The listing builds one solid part. Answer for the finished solid, in the listing's coordinates (mm). A direction names the side the tool comes from. Coordinates: 2 decimals unless noted, no trailing zeros. Order: outer loops, then holes, each group sorted by start corner. A loop starts at its lowest first (then second) coordinate and runs counter-clockwise, first axis right, second up. Notation, with made-up numbers: (44, -10) -> (89, -10) arc R25 ccw to (89, 23) -> close; hole circle Ø10 at (5, 4). An arc over 180 degrees is marked (long way). Answer in a Markdown table with one row per item.
Autodesk Inventor part; units mm, degrees
ref_plane "YZ Plane" through (0, 0, 0) normal (1, 0, 0) x (0, 1, 0)
ref_plane "XZ Plane" through (0, 0, 0) normal (0, 1, 0) x (-1, 0, 0)
ref_plane "XY Plane" through (0, 0, 0) normal (0, 0, 1) x (1, 0, 0)
sketch "Sketch1" plane through (0, 0, 0) normal (0, 0, 1) x (1, 0, 0)
  line L0 (0, 0) -> (12.5, 0)
  line L1 (12.5, 0) -> (12.5, 30)
  line L2 (12.5, 30) -> (17.5, 30)
  line L3 (17.5, 30) -> (17.5, -5)
  line L4 (17.5, -5) -> (-17.5, -5)
  line L5 (-17.5, -5) -> (-17.5, 30)
  line L6 (-17.5, 30) -> (-12.5, 30)
  line L7 (-12.5, 30) -> (-12.5, 0)
  line L8 (-12.5, 0) -> (12.5, 0)
  dimension "d0" = 12.5
  dimension "d1" = 30
  dimension "d2" = 5
  dimension "d3" = 35
  dimension "d4" = 35
  dimension "d5" = 35
  dimension "d6" = 5
  dimension "d8" = 30
extrude "Extrusion1" add sketch "Sketch1" along normal blind 10
sketch "Sketch2" plane through (-17.5, -5, 0) normal (0, -1, 0) x (1, 0, 0)
  line L0 (5, 10) -> (0, 10)
  line L1 (30, 0) -> (35, 0)
  line L2 (0, 10) -> (35, 0)
  circle A0 centre (17.5, 5) radius 3
  point P0 (17.5, 0)
  dimension "d11" = 6
extrude "Extrusion2" add sketch "Sketch2" along normal blind 50
sketch "Sketch3" plane through (-17.5, -5, 0) normal (-1, 0, 0) x (0, 0, 1)
  line L0 (0, 35) -> (10, 35)
  line L1 (5, 35) -> (5, 25)
  circle A0 centre (5, 25) radius 2.5
  point P0 (0, 5)
  dimension "d14" = 10
  dimension "d15" = 5
extrude "Extrusion3" cut sketch "Sketch3" against normal blind 35
properties part number "TopFork"
(1) A cutting plane is placed at A-A, the plane z = 5. Determine the outline of the cut face in (x, y).
Check values:
| item | result |
|---|---|
| outline | (-17.5, -5) -> (-3, -5) -> (-3, -55) -> (3, -55) -> (3, -5) -> (17.5, -5) -> (17.5, 17.5) -> (12.5, 17.5) -> (12.5, 0) -> (-12.5, 0) -> (-12.5, 17.5) -> (-17.5, 17.5) -> close; (-17.5, 22.5) -> (-12.5, 22.5) -> (-12.5, 30) -> (-17.5, 30) -> close; (12.5, 22.5) -> (17.5, 22.5) -> (17.5, 30) -> (12.5, 30) -> close |
(2) Find the intervals of material crossed by line 1 along X through (y, z) = (1, 7.25); line 2 along Y through (x, z) = (-13.75, 5); line 3 along Z through (x, y) = (13.5, 20), in increasing order. Write a range as from..to.
Check values:
| item | result |
|---|---|
| line 1 | -17.5..-12.5, 12.5..17.5 |
| line 2 | -5..17.5, 22.5..30 |
| line 3 | 0..2.5, 7.5..10 |
(3) For a pull along X with two mould halves and no side action, classify faces 1 (the flat face through (-17.5, 12, 5)), 2 (the cylindrical face through (-15.04, 22.11, 6.34)), 3 (the flat face through (-12.5, 15, 5)), 4 (the cylindrical face through (0, -30, 2)) as released by +X, released by -X, zero draft, split by the parting line, or undercut.
Check values:
| item | result |
|---|---|
| face 1 | released by -X |
| face 2 | zero draft |
| face 3 | undercut |
| face 4 | split by the parting line |
(4) A cutting plane is placed at C-C, the plane z = 1.25. Determine the outline of the cut face in (x, y).
Check values:
| item | result |
|---|---|
| outline | (-17.5, -5) -> (17.5, -5) -> (17.5, 30) -> (12.5, 30) -> (12.5, 0) -> (-12.5, 0) -> (-12.5, 30) -> (-17.5, 30) -> close |
(5) A cutting plane is placed at D-D, the plane x = 0. Determine the outline of the cut face in (y, z), then the cut area to 3 significant figures.
Check values:
| item | result |
|---|---|
| outline | (-55, 2) -> (-5, 2) -> (-5, 0) -> (0, 0) -> (0, 10) -> (-5, 10) -> (-5, 8) -> (-55, 8) -> close |
| area | 350 mm² |
(6) A cutting plane is placed at B-B, the plane y = 20. Determine the outline of the cut face in (x, z).
Check values:
| item | result |
|---|---|
| outline | (-17.5, 0) -> (-12.5, 0) -> (-12.5, 2.5) -> (-17.5, 2.5) -> close; (-17.5, 7.5) -> (-12.5, 7.5) -> (-12.5, 10) -> (-17.5, 10) -> close; (12.5, 0) -> (17.5, 0) -> (17.5, 2.5) -> (12.5, 2.5) -> close; (12.5, 7.5) -> (17.5, 7.5) -> (17.5, 10) -> (12.5, 10) -> close |
(7) Flat-ended cylindrical pins translate along their axes: pin 1 (1.5 mm diameter, centred on y = -35, z = 5.5, fed in from -X); pin 2 (4.5 mm diameter, centred on y = 20, z = 5, fed in from +X); pin 3 (5 mm diameter, centred on x = 2, z = 3, fed in from +Y); pin 4 (4 mm diameter, centred on x = 4, y = -22, fed in from +Z). Find the tip coordinate at first contact, or state that the pin passes through.
Check values:
| item | result |
|---|---|
| pin 1 | x = -3 |
| pin 2 | through |
| pin 3 | y = 0 |
| pin 4 | z = 7.24 |
(8) Which of the six approach directions +Z, -Z, +X, -X, +Y, -Y give full straight-line access (tool end or side, diameter ignored) to faces 5 (the flat face through (0, 0, 5)), 6 (the flat face through (15, 30, 5))?
Check values:
| item | result |
|---|---|
| face 5 | +Z, -Z, +Y |
| face 6 | +Z, -Z, +X, -X, +Y |
